CAD build for the part. Positions are in the model's coordinates, mm. Give positions to 0.01 mm unless a question says otherwise; leave off trailing zeros. Loops run counter-clockwise (first coordinate to the right, second up) from the corner with the lowest first, then second, coordinate; pieces in that order, holes last. Notation, with made-up numbers: (-1.5, 13.5) - (15.5, 13.5) arc R10 cw to (15.5, 17.5) - close; hole circle Ø6 at (27.25, -37). An arc over 180 degrees is marked (long way). Return JSON: item names as keys, results as strings.
from build123d import *

# Parameters (mm, degrees)
SKETCH1_W           = 240
SKETCH1_H           = 20
SKETCH1_R           = 2.5
BOSS_EXTRUDE1_DEPTH = 10
FILLET1_START       = -1
FILLET1_DEPTH       = 22


with BuildPart() as part:
    # Sketch1 → Boss-Extrude1 (new body)
    with BuildSketch(Plane.XY):
        with Locations((120, 10)):
            Rectangle(SKETCH1_W, SKETCH1_H)
        with Locations((230, 10)):
            Circle(SKETCH1_R, mode=Mode.SUBTRACT)
        with Locations((10, 10)):
            Circle(SKETCH1_R, mode=Mode.SUBTRACT)
    extrude(amount=BOSS_EXTRUDE1_DEPTH)

    # Fillet1: read off the stored shape, not the designer's step
    # Fillet1 outline → Fillet1 (cut)
    with BuildSketch(Plane(origin=(0, 0, 0), x_dir=(1, 0, 0), z_dir=(0, 1, 0)).offset(FILLET1_START)):
        with BuildLine():
            Line((0, -10), (10, -10))
            ThreePointArc((10, -10), (2.928932188, -7.071067812), (0, 0))
            Line((0, 0), (0, -10))
        make_face()
        with BuildLine():
            ThreePointArc((240, 0), (237.071067812, -7.071067812), (230, -10))
            Line((230, -10), (240, -10))
            Line((240, -10), (240, 0))
        make_face()
    extrude(amount=FILLET1_DEPTH, mode=Mode.SUBTRACT)


solid = part.part
1. Drill centre lines: probe 1 along X at (y, z) = (12.25, 4.5); probe 2 along X at (y, z) = (10, 5); probe 3 along Y at (x, z) = (230, 6). Where is each one in solid material? Low to high.
Values follow:
{"probe 1": "x = 1.07 to 8.91, 11.09 to 228.91, 231.09 to 238.93", "probe 2": "x = 1.34 to 7.5, 12.5 to 227.5, 232.5 to 238.66", "probe 3": "y = 0 to 7.5, 12.5 to 20"}
2. Drop flat-ended pins along their axis: P1, Ø4, axis at y = 2.5, z = 5, coming from the -X side; P2, Ø4, axis at y = 14, z = 8, coming from the -X side; P3, Ø5, axis at y = 5, z = 8, coming from the -X side. Give the stop position or say it passes through.
Values follow:
{"P1": "stops at x = 0.46", "P2": "stops at x = 2", "P3": "stops at x = 1.65"}
3. Cut at A-A, the plane y = 10. Write the cut outline in (x, z).
Values follow:
{"outline": "(0, 0) - (7.5, 0) - (7.5, 9.68) arc R10 ccw to start; (12.5, 0) - (227.5, 0) - (227.5, 10) - (12.5, 10) - close; (232.5, 0) - (240, 0) arc R10 ccw to (232.5, 9.68) - close"}
4. Pull direction Y, two halves, no side cores. Call faces 1 (the face through (118, 0, 5)), 2 (the face through (118, 20, 5)), 3 (the face through (9.46, 7.56, 4.93)): +Y half, -Y half, draft (parallel to the pull), parting line (faces both ways), or undercut.
Values follow:
{"face 1": "-Y half", "face 2": "+Y half", "face 3": "undercut"}
5. Cut at B-B, the plane z = 6.5. Write the cut outline in (x, y).
Values follow:
{"outline": "(2.4, 0) - (237.6, 0) - (237.6, 20) - (2.4, 20) - close; hole circle Ø5 at (10, 10); hole circle Ø5 at (230, 10)"}
